Read the model definition and answer for the solid it produces. Units are mm, in the model's axes. A direction names the side the tool comes from. Coordinates: 2 decimals unless noted, no trailing zeros. Order: outer loops, then holes, each group sorted by start corner. A loop starts at its lowest first (then second) coordinate and runs counter-clockwise, first axis right, second up. Notation, with made-up numbers: (3.25, -7.75) - (23.25, -7.75) arc R10 ccw to (23.25, 0.25) - close; hole circle Ø6 at (32.5, 22.25). An arc over 180 degrees is marked (long way). Use one line per item in the form item = value.
Autodesk Fusion 360 part; units mm, degrees
sketch "Szkic1" plane through (0, 0, 0) normal (0, 0, 1) x (1, 0, 0)
  circle A0 centre (0, 0) radius 11.5
  circle A1 centre (0, 0) radius 8.6
  circle A2 centre (0, 0) radius 5.5
  dimension "d1" = 23
  dimension "d2" = 17.2
  dimension "d7" = 11
extrude "Wyciągnięcie proste1" add sketch "Szkic1" along normal blind 7 contours A0
extrude "Wyciągnięcie proste2" add sketch "Szkic1" along normal blind 3 contours A1
sketch "Szkic2" plane through (0, 0, 0) normal (0, 0, 1) x (1, 0, 0)
  line L0 (13.1003, -4.95) -> (-13.365, -4.95)
  line L1 (-13.365, -4.95) -> (-13.365, 5.05)
  line L2 (-13.365, 5.05) -> (13.635, 5.05)
  line L3 (13.1003, -4.95) -> (-13.365, 5.05) construction
  line L4 (-13.365, -4.95) -> (13.635, 5.05) construction
  line L5 (35, -4.95) -> (-35, -4.95)
  line L6 (-35, -4.95) -> (-35, 4.95)
  line L7 (-35, 4.95) -> (35, 4.95)
  line L8 (35, 4.95) -> (35, -4.95)
  line L9 (35, -4.95) -> (-35, 4.95) construction
  line L10 (-13.365, -4.95) -> (-21.365, -4.95)
  line L11 (-21.365, -4.95) -> (-21.365, 4.95)
  line L12 (-21.365, 4.95) -> (-13.365, 4.95)
  line L13 (-13.365, 4.95) -> (-13.365, -4.95)
  circle A0 centre (0, 0) radius 11.5
  line L14 (-35, -4.95) -> (-11.3867, -1.6104) construction
  line L15 (0, 0) -> (35, 4.95) construction
  line L16 (-18.365, 4.95) -> (-18.365, -4.95)
  circle A1 centre (0, 0) radius 35
  circle A2 centre (-31, 0) radius 1.75
  circle A3 centre (31, 0) radius 1.75
  dimension "d8" = 27
  dimension "d9" = 10
  dimension "d10" = 70
  dimension "d11" = 9.9
  dimension "d12" = 8
  dimension "d15" = 3
  dimension "d36" = 3.5
  dimension "d37" = 4
  dimension "d38" = 4
extrude "Wyciągnięcie proste3" add sketch "Szkic2" along normal blind 7 contours L0 L5 L7 A0 A1 | L0 L1 L5 L7 L13 A0 | L5 L7 L11 A1 | L1 L5 L7 L10 L12 L13 L16 | L5 L7 L10 L11 L12 L16
(1) Which of the six approach directions +Z, -Z, +X, -X, +Y, -Y give full straight-line access (tool end or side, diameter ignored) to faces 4 (the flat face through (-22, -4.95, 3)), 5 (the flat face through (23, -4.95, 3)), 6 (the flat face through (-23, 4.95, 3)), 7 (the flat face through (22, 4.95, 3))?
Answer list:
face_4 = +Z, -Z, -X, -Y
face_5 = +Z, -Z, +X, -Y
face_6 = +Z, -Z, -X, +Y
face_7 = +Z, -Z, +X, +Y
(2) Section D-D, the plane x = 31 is taken. Write down the section's boundary in (y, z).
Answer list:
outline = (-4.95, 0) - (-1.75, 0) - (-1.75, 7) - (-4.95, 7) - close; (1.75, 0) - (4.95, 0) - (4.95, 7) - (1.75, 7) - close
(3) Given pin 1 Ø3.5 at (x, z) = (24, 5) entering from +Y; pin 2 Ø6.5 at (x, y) = (0, 0) entering from +Z; pin 3 Ø5 at (x, y) = (-3, 2.5) entering from +Z; pin 4 Ø4 at (x, z) = (-26, 4) entering from -Y, each flat-ended and moving along its own axis, determine where each tip first touches the part or whether it passes through.
Answer list:
pin_1 = 4.95
pin_2 = through
pin_3 = 3
pin_4 = -4.95
(4) Straight lines are drawn through the part: L1, parallel to X at y = -1, z = 6.5; L2, parallel to Y at x = 22.5, z = 6; L3, parallel to X at y = -0.75, z = 2.25. For each, find the intervals that lie inside material, in ascending order.
Answer list:
L1 = -34.99 to -32.44, -29.56 to -8.54, 8.54 to 29.56, 32.44 to 34.99
L2 = -4.95 to 4.95
L3 = -34.99 to -32.58, -29.42 to -5.45, 5.45 to 29.42, 32.58 to 34.99
(5) Section A-A, the plane x = 0 is taken. Write down the section's boundary in (y, z).
Answer list:
outline = (-11.5, 0) - (-5.5, 0) - (-5.5, 3) - (-8.6, 3) - (-8.6, 7) - (-11.5, 7) - close; (5.5, 0) - (11.5, 0) - (11.5, 7) - (8.6, 7) - (8.6, 3) - (5.5, 3) - close
(6) Section C-C, the plane z = 5.75 is taken. Write down the section's boundary in (x, y).
Answer list:
outline = (-34.65, -4.95) - (-10.38, -4.95) arc R11.5 ccw to (10.38, -4.95) - (34.65, -4.95) arc R35 ccw to (34.65, 4.95) - (10.38, 4.95) arc R11.5 ccw to (-10.38, 4.95) - (-34.65, 4.95) arc R35 ccw to start; hole circle Ø3.5 at (-31, 0); hole circle Ø17.2 at (0, 0); hole circle Ø3.5 at (31, 0)
(7) The mould has two halves that part along Y. Classify faces 1 (the cylindrical face through (-32.75, -0.08, 3.45)), 2 (the cylindrical face through (0.2, -11.5, 3.5)), 3 (the cylindrical face through (-35, 0, 3)): +Y half, -Y half, draft (parallel to the pull), parting line (faces both ways), or undercut.
Answer list:
face_1 = undercut
face_2 = -Y half
face_3 = parting line
(8) Section B-B, the plane y = 0 is taken. Write down the section's boundary in (x, z), then the cut area to 3 significant figures.
Answer list:
outline = (-35, 0) - (-32.75, 0) - (-32.75, 7) - (-35, 7) - close; (-29.25, 0) - (-5.5, 0) - (-5.5, 3) - (-8.6, 3) - (-8.6, 7) - (-29.25, 7) - close; (5.5, 0) - (29.25, 0) - (29.25, 7) - (8.6, 7) - (8.6, 3) - (5.5, 3) - close; (32.75, 0) - (35, 0) - (35, 7) - (32.75, 7) - close
area = 339 mm2
